Autodesk Inventor part; units mm, degrees
ref_plane "YZ Plane" through (0, 0, 0) normal (1, 0, 0) x (0, 1, 0)
ref_plane "XZ Plane" through (0, 0, 0) normal (0, 1, 0) x (-1, 0, 0)
ref_plane "XY Plane" through (0, 0, 0) normal (0, 0, 1) x (1, 0, 0)
sketch "Sketch1" plane through (0, 0, 0) normal (0, 1, 0) x (-1, 0, 0)
  line L0 (-50, 115) -> (50, 115)
  line L1 (50, 115) -> (50, -115)
  line L2 (50, -115) -> (-50, -115)
  line L3 (-50, -115) -> (-50, 115)
  line L4 (-50, 115) -> (50, -115) construction
  line L5 (50, 115) -> (-50, -115) construction
  circle A0 centre (0, -65) radius 43.5
  circle A1 centre (0, -65) radius 36
  line L6 (-28.75, 100) -> (28.75, 100)
  line L7 (28.75, 100) -> (28.75, 39.5)
  line L8 (28.75, 39.5) -> (-28.75, 39.5)
  line L9 (-28.75, 39.5) -> (-28.75, 100)
  line L10 (-28.75, 100) -> (28.75, 39.5) construction
  line L11 (28.75, 100) -> (-28.75, 39.5) construction
  point P0 (0, 0)
  point P1 (0, 69.75)
  dimension "d0" = 7.5
  dimension "d1" = 72
  dimension "d2" = 60.5
  dimension "d3" = 57.5
  dimension "d4" = 100
  dimension "d5" = 230
  dimension "d6" = 15
  dimension "d7" = 50
extrude "Extrusion1" add sketch "Sketch1" along normal blind 8
extrude "Extrusion2" add sketch "Sketch1" along normal blind 5 contours A0
sketch "Sketch2" plane through (0, 0, 0) normal (0, -1, 0) x (1, 0, 0)
  line L0 (50, -115) -> (-50, -115)
  line L1 (50, 115) -> (50, -115)
  line L2 (-50, 115) -> (50, 115)
  line L3 (-50, -115) -> (-50, 115)
  line L4 (28.75, 100) -> (-28.75, 100)
  line L5 (28.75, 39.5) -> (28.75, 100)
  line L6 (-28.75, 39.5) -> (28.75, 39.5)
  line L7 (-28.75, 100) -> (-28.75, 39.5)
  line L8 (-36.25, 37.25) -> (32.75, 37.25)
  line L9 (32.75, 37.25) -> (32.75, 102.25)
  line L10 (32.75, 102.25) -> (-36.25, 102.25)
  line L11 (-36.25, 102.25) -> (-36.25, 37.25)
  line L12 (-36.25, 37.25) -> (32.75, 102.25) construction
  line L13 (32.75, 37.25) -> (-36.25, 102.25) construction
  point P0 (0, 0)
  point P1 (-1.75, 69.75)
  dimension "d12" = 69
  dimension "d13" = 65
  dimension "d14" = 4
  dimension "d15" = 2.25
extrude "Extrusion3" cut sketch "Sketch2" against normal blind 3 contours L11 L10 L9 L8
sketch "Sketch3" plane through (0, 5, -65) normal (0, 1, 0) x (1, 0, 0)
  circle A0 centre (0, 0) radius 36
  circle A1 centre (0, 0) radius 43.5
  circle A2 centre (0, 0) radius 43.5
  circle A3 centre (0, 0) radius 36
  circle A4 centre (0, 0) radius 36
  line L0 (50, 50) -> (-50, 50)
  line L1 (-50, 50) -> (-50, -180)
  line L2 (-50, -180) -> (50, -180)
  line L3 (50, -180) -> (50, 50)
  line L4 (28.75, -165) -> (-28.75, -165)
  line L5 (-28.75, -165) -> (-28.75, -104.5)
  line L6 (-28.75, -104.5) -> (28.75, -104.5)
  line L7 (28.75, -104.5) -> (28.75, -165)
  circle A5 centre (0, 0) radius 43.5
  line L8 (-35.2101, 7.5) -> (-42.8486, 7.5)
  line L9 (-42.8486, -7.5) -> (-35.2101, -7.5)
  point P0 (0, -65)
  point P1 (-39.0293, -7.5)
  point P2 (-35.2101, 7.5)
  point P3 (-42.8486, 7.5)
  dimension "d18" = 15
extrude "Extrusion4" cut sketch "Sketch3" against normal through all contours A0 L9 A1 L8 picked at (-37.9902, -5.8388)
sketch "Sketch4" plane through (0, 0, 0) normal (0, -1, 0) x (1, 0, 0)
  arc A0 (-35.2101, -72.5) -> (-35.2101, -57.5) centre (0, -65) ccw
  arc A1 (-42.8486, -72.5) -> (-42.8486, -57.5) centre (0, -65) ccw
  line L0 (-31, -44.5) -> (31, -44.5)
  line L1 (31, -44.5) -> (31, -85.5)
  line L2 (31, -85.5) -> (-31, -85.5)
  line L3 (-31, -85.5) -> (-31, -44.5)
  line L4 (-31, -44.5) -> (31, -85.5) construction
  line L5 (31, -44.5) -> (-31, -85.5) construction
  point P0 (0, 0)
  point P1 (-31, -46.697)
  point P2 (-31, -83.303)
  point P3 (-29.5931, -85.5)
  point P4 (29.5931, -85.5)
  point P5 (31, -83.303)
  point P6 (31, -46.697)
  point P7 (29.5931, -44.5)
  point P8 (-29.5931, -44.5)
  dimension "d21" = 41
  dimension "d22" = 62
extrude "Extrusion5" cut sketch "Sketch4" against normal blind 2 contours L3 A0 L0 L1 L2 | A0 L2 L3 | L3 L0 A0 | A0 L1 L2 | L0 L1 A0
sketch "Sketch5" plane through (0, 2, 0) normal (0, -1, 0) x (1, 0, 0)
  line L0 (-31, -85.5) -> (-31, -44.5)
  line L1 (-31, -46.697) -> (-23, -46.697)
  line L2 (-23, -46.697) -> (-23, -83.303)
  line L3 (-23, -83.303) -> (-31, -83.303)
  line L4 (-31, -83.303) -> (-31, -46.697)
  point P0 (0, 0)
  point P1 (-27, -83.303)
  dimension "d25" = 8
extrude "Extrusion6" cut sketch "Sketch5" against normal blind 1
sketch "Sketch6" plane through (0, 0, 0) normal (0, -1, 0) x (1, 0, 0)
  circle A0 centre (25.4, -28.375) radius 1.25
  circle A1 centre (26.7, 20.625) radius 1.25
  circle A2 centre (-24.8, 15.525) radius 1.25
  circle A3 centre (-24.8, -13.375) radius 1.25
  line L0 (-31, -44.5) -> (31, -44.5)
  line L1 (32.75, 37.25) -> (-36.25, 37.25)
  point P0 (0, 0)
  point P1 (25.4, -3.625)
  point P2 (-29.5931, -44.5)
  point P3 (29.5931, -44.5)
  dimension "d28" = 2.5
  dimension "d29" = 2.5
  dimension "d30" = 2.5
  dimension "d31" = 2.5
  dimension "d32" = -28.9
  dimension "d33" = -1.3
  dimension "d34" = -51.5
  dimension "d35" = -49
  dimension "d36" = -5.1
  dimension "d37" = -24.75
  dimension "d38" = 81.75
  dimension "d64" = 40.875
extrude "Extrusion7" add sketch "Sketch6" along normal blind 5
sketch "Sketch7" plane through (0, 0, 0) normal (0, -1, 0) x (1, 0, 0)
  line L0 (-36.25, 37.25) -> (-36.25, 102.25)
  line L1 (-36.25, 96.25) -> (-42.25, 96.25)
  line L2 (-42.25, 96.25) -> (-42.25, 43.25)
  line L3 (-42.25, 43.25) -> (-36.25, 43.25)
  line L4 (-36.25, 43.25) -> (-36.25, 96.25)
  line L5 (-36.25, 102.25) -> (32.75, 102.25)
  line L6 (32.75, 37.25) -> (-36.25, 37.25)
  point P0 (0, 0)
  point P1 (-39.25, 96.25)
  point P2 (-39.25, 43.25)
  dimension "d43" = 6
  dimension "d44" = 6
  dimension "d45" = 6
extrude "Extrusion8" cut sketch "Sketch7" against normal up to surface (3 mm away)
sketch "Sketch8" plane through (50, 0, -115) normal (0, 0, -1) x (-1, 0, 0)
  line L0 (0, 0) -> (100, 0)
  line L1 (100, 0) -> (100, 8)
  line L2 (100, 0) -> (93.0541, -39.3923)
  line L3 (93.0541, -39.3923) -> (83.206, -37.6558)
  line L4 (83.206, -37.6558) -> (89.8457, 0)
  line L5 (100, 0) -> (101.4106, 8)
  line L6 (101.4106, 8) -> (100, 8)
  point P0 (50, 0)
  dimension "d65" = 10
  dimension "d66" = 80
  dimension "d67" = 170
  dimension "d68" = 48.1234
  dimension "d69" = 40
  dimension "d70" = 80
  dimension "d71" = 38.2367
extrude "Extrusion9" add sketch "Sketch8" against normal blind 10
sketch "Sketch9" plane through (-50, 0, 115) normal (0, 0, 1) x (1, 0, 0)
  line L0 (0, 0) -> (10.1543, 0)
  line L1 (101.4106, 8) -> (100, 8)
  line L2 (100, 0) -> (100, 8)
  line L3 (100, 0) -> (101.4106, 8)
  line L4 (0, 0) -> (6.9459, -39.3923)
  line L5 (6.9459, -39.3923) -> (16.794, -37.6558)
  line L6 (16.794, -37.6558) -> (10.1543, 0)
  line L7 (0, 8) -> (-1.4106, 8)
  line L8 (-1.4106, 8) -> (0, 0)
  line L9 (0, 8) -> (0, 0)
  point P0 (50, 0)
extrude "Extrusion10" add sketch "Sketch9" against normal blind 10 contours L0 L6 L5 L4 | L8 L7 L9
sketch "Sketch10" plane through (0, 8, 0) normal (0, 1, 0) x (1, 0, 0)
  circle A0 centre (39.375, -69.75) radius 3.25
  line L0 (28.75, -39.5) -> (28.75, -100)
  line L1 (50, -115) -> (50, 115)
  point P0 (0, 0)
  point P1 (28.75, -69.75)
  point P2 (50, -105)
  point P3 (50, 105)
  dimension "d56" = 6.5
  dimension "d57" = 21.25
  dimension "d58" = 10.625
extrude "Extrusion11" cut sketch "Sketch10" against normal through all
sketch "Sketch11" plane through (0, 0, 0) normal (0, -1, 0) x (1, 0, 0)
  circle A0 centre (39.375, 69.75) radius 3.25
  circle A1 centre (39.375, 69.75) radius 5
  point P0 (0, 0)
  dimension "d61" = 10
extrude "Extrusion12" cut sketch "Sketch11" against normal blind 4.5 contours A0 | A1
properties part number "ViesCooleHouder"
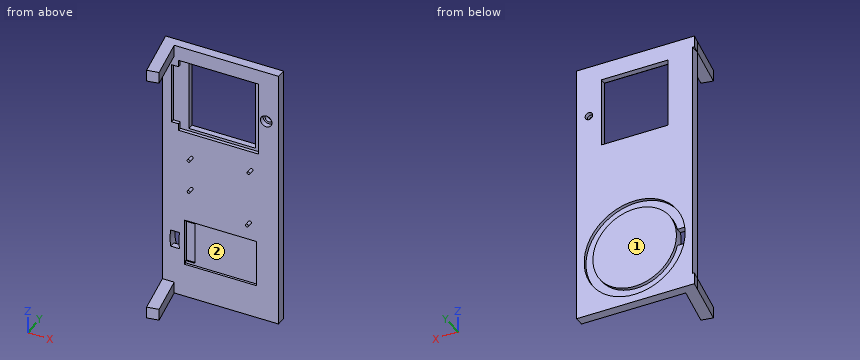
The listing builds one solid part. Answer for the finished solid, in the listing's coordinates (mm). Face numbers are marked on the shaded views. Give positions to 0.01 mm unless a question says otherwise; leave off trailing zeros. Order: outer loops, then holes, each group sorted by start corner. A loop starts at its lowest first (then second) coordinate and runs counter-clockwise, first axis right, second up. Notation, with made-up numbers: (70.5, 66) - (103.5, 66) arc R18 cw to (103.5, 99) - close; hole circle Ø8 at (43, -3). An arc over 180 degrees is marked (long way). Use one line per item in the form item = value.
1) Each of these flat-tipped pins is pushed along its axis until it touches: pin 1 (0.8 mm diameter, centred on x = 25, z = -28.5, fed in from -Y); pin 2 (6.5 mm diameter, centred on x = -26.5, z = -68, fed in from -Y); pin 3 (4 mm diameter, centred on x = 34.5, z = 78.5, fed in from -Y). Where does it stop, or does it pass through?
Verdict:
pin_1 = -5
pin_2 = 3
pin_3 = 0
2) The mould has two halves that part along Z. Classify the marked faces 1 and 2: released by +Z, released by -Z, zero draft, split by the parting line, or undercut.
Verdict:
face_1 = zero draft
face_2 = undercut
3) Consider probe 1 along X at (y, z) = (7, 69.75) (3 decimals); probe 2 along X at (y, z) = (5, 69); probe 3 along X at (y, z) = (4.75, -65). Determine where each line is inside the solid, lowest interval first. Write a range as [from, to].
Verdict:
probe_1 = [-50, -28.75], [28.75, 36.125], [42.625, 50]
probe_2 = [-50, -28.75], [28.75, 36.21], [42.54, 50]
probe_3 = [-50, -43.5], [-36, 50]
4) Find section C-C on y = -19. Determine the outline of the cut face in (x, z), and give its area (3 significant figures).
Verdict:
outline = (-46.65, -115) - (-36.5, -115) - (-36.5, -105) - (-46.65, -105) - close; (-46.65, 105) - (-36.5, 105) - (-36.5, 115) - (-46.65, 115) - close
area = 203 mm^2
5) Find section D-D on z = 27. Determine the outline of the cut face in (x, y), and give its area (3 significant figures).
Verdict:
outline = (-50, 0) - (50, 0) - (50, 8) - (-50, 8) - close
area = 800 mm^2
6) Find section B-B on x = 12. Determine the outline of the cut face in (y, z), and give its area (3 significant figures).
Verdict:
outline = (0, -115) - (8, -115) - (8, -106.81) - (5, -106.81) - (5, -98.94) - (8, -98.94) - (8, -31.06) - (5, -31.06) - (5, -23.19) - (8, -23.19) - (8, 39.5) - (3, 39.5) - (3, 37.25) - (0, 37.25) - (0, -44.5) - (2, -44.5) - (2, -85.5) - (0, -85.5) - close; (0, 102.25) - (3, 102.25) - (3, 100) - (8, 100) - (8, 115) - (0, 115) - close
area = 1,210 mm^2
7) Find section A-A on z = -65. Determine the outline of the cut face in (x, y).
Verdict:
outline = (-50, 0) - (-43.5, 0) - (-43.5, 8) - (-50, 8) - close; (-36, 0) - (-31, 0) - (-31, 3) - (-23, 3) - (-23, 2) - (31, 2) - (31, 0) - (50, 0) - (50, 8) - (43.5, 8) - (43.5, 5) - (36, 5) - (36, 8) - (-36, 8) - close
